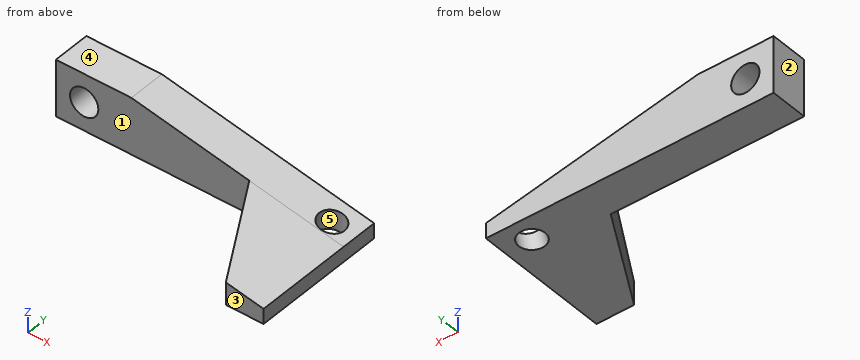
```python
from build123d import *

# Parameters (mm, degrees)
F0_R     = 1.5
F1_DEPTH = 4
F3_DEPTH = 10.5
F5_DEPTH = 6.001
F6_R     = 1.375
F7_DEPTH = 7.424825


with BuildPart() as f1:
    # F0 (on Front) → F1 (new body)
    with BuildSketch(Plane.XZ):
        Polygon((5, 3), (-3, 3), (-3, -3), (27.5, -3), (27.5, -1.4), align=None)
        Circle(F0_R, mode=Mode.SUBTRACT)
    extrude(amount=F1_DEPTH)

    # F2 (on face) → F3 (join)
    with BuildSketch(Plane.XZ.offset(4)):
        Polygon((17.5, -3), (27.5, -3), (27.5, -1.4), (17.5, 0.555556), align=None)
    extrude(amount=F3_DEPTH)

    # F4 (on face) → F5 (cut, through all)
    with BuildSketch(Plane(origin=(0, 0, -3), x_dir=(1, 0, 0), z_dir=(0, 0, -1))):
        Polygon((23.5, 14.5), (17.5, 14.5), (17.5, 4), align=None)
    extrude(amount=-F5_DEPTH, mode=Mode.SUBTRACT)

    # F6 (on face) → F7 (cut, through all)
    with BuildSketch(Plane(origin=(0.749225, 0, 3.831263), x_dir=(0.981411, 0, -0.19192), z_dir=(0.19192, 0, 0.981411))):
        with Locations((24.757478, -2.5)):
            Circle(F6_R)
    extrude(amount=-F7_DEPTH, mode=Mode.SUBTRACT)


solid = f1.part
```
Design review of the part built by this model. Coordinates are the model's own, in mm. Face numbers are marked on the shaded views. A direction names the side the tool comes from. Round coordinates to 2 decimals unless told otherwise and drop trailing zeros. Order: outer loops, then holes, each group sorted by start corner. A loop starts at its lowest first (then second) coordinate and runs counter-clockwise, first axis right, second up. Notation, with made-up numbers: (-27.75, -3.75) - (13.25, -3.75) arc R24 ccw to (13.25, 10.25) - close; hole circle Ø9 at (64.25, -28.75). An arc over 180 degrees is marked (long way). Return JSON: item names as keys, results as strings.
Q1. Consider section C-C on z = 0.9. Write out the cut boundary in (x, y).
Computed values:
{"outline": "(-3, -4) - (-1.2, -4) - (-1.2, 0) - (-3, 0) - close; (1.2, -4) - (15.74, -4) - (15.74, 0) - (1.2, 0) - close"}
Q2. Machinability: for the marked faces 1 and 2, which of the approach directions +Z, -Z, +X, -X, +Y, -Y give a long, thin tool a straight path to every point of the face, cutting with its end or side? Answer none if there is none.
Computed values:
{"face 1": "+Z, -Z, -X, -Y", "face 2": "+Z, -Z, -X, +Y, -Y"}
Q3. Wall thickness on L1, parallel to Z at x = 0, y = -1.75; L2, parallel to Y at x = 11, z = 0.05; L3, parallel to Z at x = 25, y = -7.5: over which ranges is each line inside the solid? List them lowest first. Write a range as [from, to].
Computed values:
{"L1": "z = [-3, -1.5], [1.5, 3]", "L2": "y = [-4, 0]", "L3": "z = [-3, -0.91]"}
Q4. Consider section D-D on y = -5.75. Write out the cut boundary in (x, z).
Computed values:
{"outline": "(18.5, -3) - (27.5, -3) - (27.5, -1.4) - (18.5, 0.36) - close"}
Q5. Consider section A-A on x = 0. Write out the cut boundary in (y, z), plus the area to 3 significant figures.
Computed values:
{"outline": "(-4, -3) - (0, -3) - (0, -1.5) - (-4, -1.5) - close; (-4, 1.5) - (0, 1.5) - (0, 3) - (-4, 3) - close", "area": "12.0 mm2"}
Q6. The part is to be moulded in two halves that separate along Y. For the marked faces 3, 4 and 5, say which applies: pulls with the +Y half, pulls with the -Y half, needs draft (parallel to the pull), parting line crosses it, or undercut.
Computed values:
{"face 3": "pulls with the -Y half", "face 4": "needs draft", "face 5": "undercut"}
Q7. For pin 1 Ø6 at (x, y) = (19, -4.5) entering from +Z, flat-tipped, find the tip position at first contact; note if it passes through.
Computed values:
{"pin 1": "stops at z = 0.84"}
Q8. Consider section B-B on y = -3.5. Write out the cut boundary in (x, z), plus the area to 3 significant figures.
Computed values:
{"outline": "(-3, -3) - (23.68, -3) - (24.12, -0.74) - (5, 3) - (-3, 3) - close; (25.6, -3) - (27.5, -3) - (27.5, -1.4) - (25.97, -1.1) - close; hole circle Ø3 at (0, 0)", "area": "122 mm2"}
